Read the model definition and answer for the solid it produces. Units are mm, in the model's axes. Face numbers are marked on the shaded views. A direction names the side the tool comes from. Round coordinates to 2 decimals unless told otherwise and drop trailing zeros. Loops run counter-clockwise (first coordinate to the right, second up) from the corner with the lowest first, then second, coordinate; pieces in that order, holes last. Notation, with made-up numbers: (83.5, 88) - (101.5, 88) arc R28 cw to (101.5, 123) - close; hole circle Ø5 at (16, 51). An arc over 180 degrees is marked (long way). Use one line per item in the form item = value. Start each with the question number.
Autodesk Inventor part; units mm, degrees
ref_plane "YZ Plane" through (0, 0, 0) normal (1, 0, 0) x (0, 1, 0)
ref_plane "XZ Plane" through (0, 0, 0) normal (0, 1, 0) x (-1, 0, 0)
ref_plane "XY Plane" through (0, 0, 0) normal (0, 0, 1) x (1, 0, 0)
sketch "Sketch1" plane through (0, 0, 0) normal (0, 1, 0) x (-1, 0, 0)
  line L0 (15, 5) -> (-15, 5)
  line L1 (-15, 5) -> (-15, -5)
  line L2 (-15, -5) -> (15, -5)
  line L3 (15, -5) -> (15, 5)
  point P0 (0, 0)
  point P1 (15, 0)
  point P2 (0, 5)
  dimension "d0" = 30
  dimension "d1" = 10
extrude "Extrusion1" add sketch "Sketch1" along normal blind 5
sketch "Sketch3" plane through (0, 5, 0) normal (0, 1, 0) x (1, 0, 0)
  line L0 (-15, -5) -> (15, -5)
  line L1 (-6, 5) -> (6, 5)
  line L2 (6, 5) -> (6, -5)
  line L3 (6, -5) -> (-6, -5)
  line L4 (-6, -5) -> (-6, 5)
  line L5 (15, 5) -> (-15, 5)
  point P0 (0, 0)
  point P1 (0, 5)
  dimension "d13" = 12
  dimension "d14" = 6
extrude "Extrusion2" add sketch "Sketch3" along normal blind 7
sketch "Sketch4" plane through (-15, 0, 5) normal (0, 0, 1) x (1, 0, 0)
  line L0 (9, 12) -> (21, 12)
  line L1 (9, 5) -> (9, 12)
  line L2 (0, 5) -> (9, 5)
  line L3 (0, 0) -> (30, 0)
  point P0 (15, 0)
  point P1 (15, 5)
  dimension "d18" = 6
  dimension "d45" = 5
hole "Hole2" at (0, 5, 5) direction (0, 0, -1) diameter 6 end through all
sketch "Sketch5" plane through (-15, 0, 5) normal (0, 0, 1) x (1, 0, 0)
  line L0 (9, 12) -> (21, 12)
  line L1 (21, 5) -> (21, 12)
  line L2 (0, 5) -> (9, 5)
  line L3 (0, 0) -> (30, 0)
  line L4 (19.8497, 5) -> (17.4249, 0.8)
  line L5 (17.4249, 0.8) -> (12.5751, 0.8)
  line L6 (12.5751, 0.8) -> (10.1503, 5)
  line L7 (10.1503, 5) -> (12.5751, 9.2)
  line L8 (12.5751, 9.2) -> (17.4249, 9.2)
  line L9 (17.4249, 9.2) -> (19.8497, 5)
  point P0 (15, 0)
  point P1 (15, 5)
  point P2 (13.175, 20)
  point P3 (16.825, 20)
  point P4 (20, 13.175)
  point P5 (20, 16.825)
  point P6 (15, 5)
  dimension "d46" = 5
  dimension "d47" = 8.4
  dimension "d48" = 6
extrude "Extrusion3" cut sketch "Sketch5" against normal blind 5
fillet "Fillet2" radius 6 2 edges at (-6, 12, 0) (6, 12, 0)
fillet "Fillet3" radius 2.5 2 edges at (6, 5, 0) (-6, 5, 0)
sketch "Sketch6" plane through (0, 0, 0) normal (0, -1, 0) x (1, 0, 0)
  line L0 (-15, -5) -> (-15, 5)
  line L1 (15, 5) -> (15, -5)
  point P0 (0, 0)
  point P1 (-11, 0)
  point P2 (11, 0)
  dimension "d33" = 4
  dimension "d34" = 4
hole "Hole3" at (-11, 0, 0) at (11, 0, 0) direction (0, 1, 0) diameter 3 end through all
properties part number "motor_bracket"
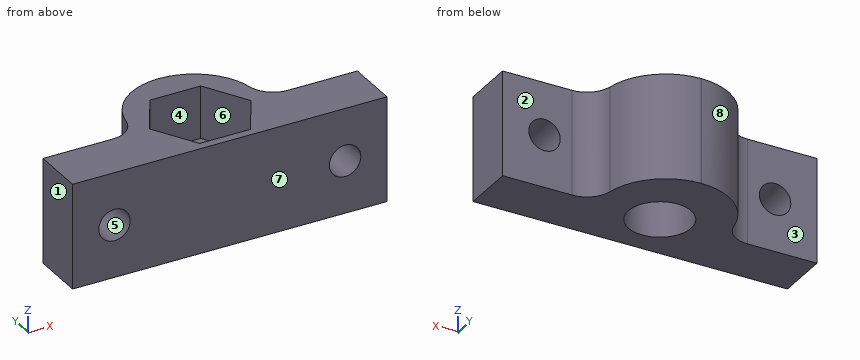
1) Determine the mould class of the marked faces 6, 7 and 8 for opening direction X: +X half, -X half, draft (parallel to the pull), parting line (faces both ways), or undercut.
2) Straight lines are drawn through the part: line 1 (Z direction, x = -11, y = 2.3); line 2 (Y direction, x = 0, z = -1.2); line 3 (Y direction, x = -13.5, z = -2). For each, find the intervals that lie inside material, in ascending order. Write a range as from..to.
3) A cutting plane is placed at A-A on y = 2.5. Write down the section's boundary in (x, z), plus the area to 3 significant figures.
4) A cutting plane is placed at C-C on z = 0.5. Count the separate pieces of the cut face and the enclosed holes in it, plus the area to 3 significant figures.
5) For the marked faces 1, 2, 3, 4 and 5, determine the directions among +Z, -Z, +X, -X, +Y, -Y from which every point of the face is accessible in a straight line to the end or side of a thin tool.
6) Flat-ended cylindrical pins translate along their axes: pin 1 (5.5 mm diameter, centred on x = -13, z = 1.5, fed in from +Y); pin 2 (7 mm diameter, centred on x = 0, y = 5, fed in from +Z); pin 3 (1.5 mm diameter, centred on x = -1, z = 3, fed in from +Y); pin 4 (2.5 mm diameter, centred on x = 11, z = 0, fed in from +Y). Find the tip coordinate at first contact, or state that the pin passes through.
7) A cutting plane is placed at B-B on x = -11. Write down the section's boundary in (y, z), plus the area to 3 significant figures.
8) A cutting plane is placed at D-D on x = 0.5. Write down the section's boundary in (y, z), plus the area to 3 significant figures.
Checks:
q1.face_6 = undercut
q1.face_7 = draft
q1.face_8 = -X half
q2.line_1 = -5..-1.5, 1.5..5
q2.line_2 = 0..2, 8..12
q2.line_3 = 0..5
q3.outline = (-15, -5) - (-1.66, -5) - (-1.66, 0) - (-3.41, 0) - (-3.41, 5) - (-15, 5) - close; (1.66, -5) - (15, -5) - (15, 5) - (3.41, 5) - (3.41, 0) - (1.66, 0) - close; hole circle Ø3 at (-11, 0); hole circle Ø3 at (11, 0)
q3.area = 235 mm²
q4.separate_pieces = 3
q4.enclosed_holes = 1
q4.area = 131 mm²
q5.face_1 = +Z, -Z, -X, +Y, -Y
q5.face_2 = +Z, -Z, +X, +Y
q5.face_3 = +Z, -Z, -X, +Y
q5.face_4 = +Z
q5.face_5 = +Y, -Y
q6.pin_1 = 5
q6.pin_2 = 0
q6.pin_3 = 11.99
q6.pin_4 = through
q7.outline = (0, -5) - (5, -5) - (5, -1.5) - (0, -1.5) - close; (0, 1.5) - (5, 1.5) - (5, 5) - (0, 5) - close
q7.area = 35.0 mm²
q8.outline = (0, -5) - (2.04, -5) - (2.04, 0) - (0.8, 0) - (0.8, 5) - (0, 5) - close; (7.96, -5) - (11.98, -5) - (11.98, 5) - (9.2, 5) - (9.2, 0) - (7.96, 0) - close
q8.area = 48.2 mm²
